Can you work these out from the drawing? Everything is in mm from the part's minimum corner. A direction names the side the tool comes from. Round coordinates to 2 decimals unless told otherwise and drop trailing zeros. Write each loop counter-clockwise with the first axis right and the second up, starting at its lowest first coordinate (ties: lowest second). Pieces come first, ordered by that corner, then holes. Notation, with made-up numbers: (15, -13) -> (25, -13) arc R23 cw to (25, 17) -> close; hole circle Ø1 at (21.5, 15.25). An arc over 180 degrees is marked (long way). Answer as CSV lines item,"result". Start each with the question number.
Q1. Imagine slicing it at B-B on z = 6. Please give me the cut outline in (x, y), and give its area (3 significant figures).
Q2. If I drill on line 1 (Y direction, x = 3.5, z = 55); line 2 (Y direction, x = 10.75, z = 39); line 3 (Z direction, x = 23, y = 32.5), over which ranges is the centre line in solid material (lowest first)? Write a range as [from, to].
Q3. Imagine slicing it at C-C on y = 28. Please give me the cut outline in (x, z), and give its area (3 significant figures).
Q4. For the marked faces 1 and 2, which set-ups out of +Z, -Z, +X, -X, +Y, -Y let a thin tool reach every point of the face, with its end or its side?
Q5. Imagine slicing it at A-A on x = 15.75. Please give me the cut outline in (y, z), and give its area (3 significant figures).
Q6. Will these pins go through, and if not, where does the flat tip stop? pin 1 Ø10 at (x, y) = (2.5, 33) entering from +Z; pin 2 Ø6 at (x, z) = (8.5, 52.5) entering from +Y; pin 3 Ø4 at (x, z) = (2.5, 39) entering from +Y.
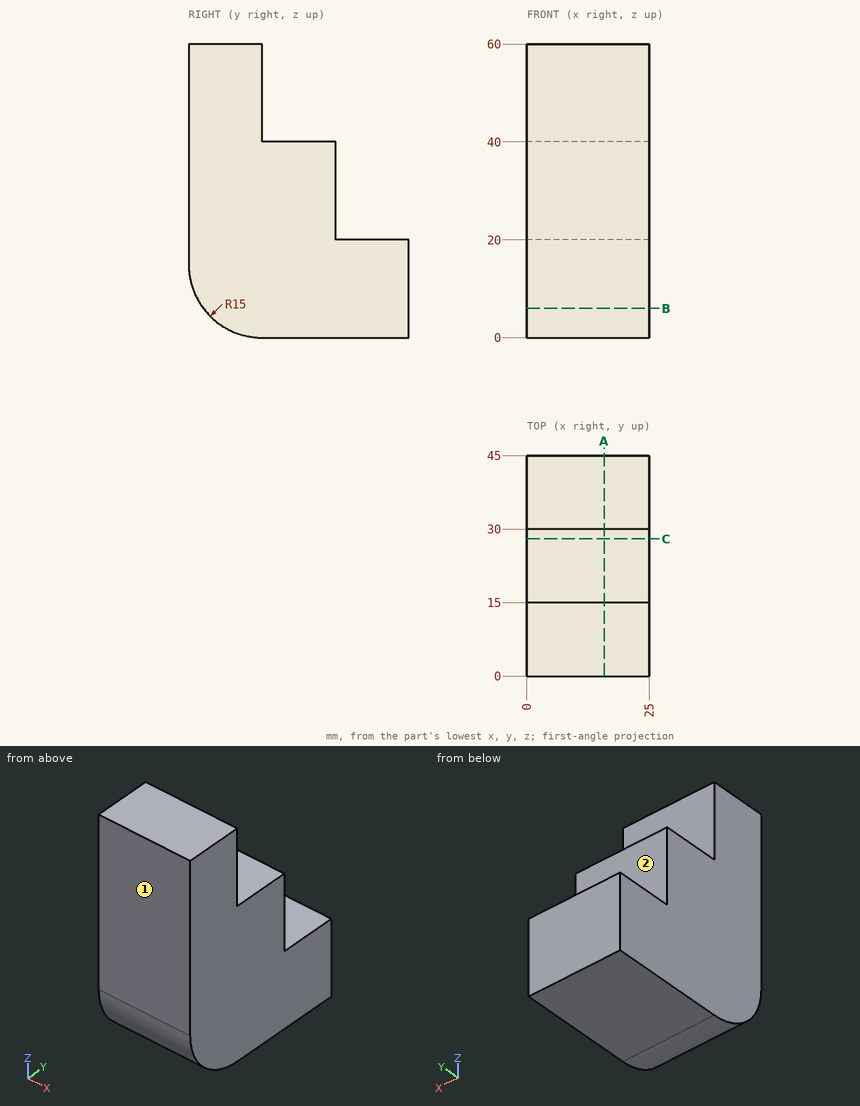
Checks:
1,outline,"(0, 3) -> (25, 3) -> (25, 45) -> (0, 45) -> close"
1,area,"1,050 mm^2"
2,line 1,"[0, 15]"
2,line 2,"[0, 30]"
2,line 3,"[0, 20]"
3,outline,"(0, 0) -> (25, 0) -> (25, 40) -> (0, 40) -> close"
3,area,"1,000 mm^2"
4,face 1,"+Z, -Z, +X, -X, -Y"
4,face 2,"+Z, +X, -X, +Y"
5,outline,"(0, 15) arc R15 ccw to (15, 0) -> (45, 0) -> (45, 20) -> (30, 20) -> (30, 40) -> (15, 40) -> (15, 60) -> (0, 60) -> close"
5,area,"1,750 mm^2"
6,pin 1,"z = 40"
6,pin 2,"y = 15"
6,pin 3,"y = 30"
